For this review, take the finished solid that the model builds, in its own axes (mm). Face numbers are marked on the shaded views. A direction names the side the tool comes from. Round coordinates to 2 decimals unless told otherwise and drop trailing zeros. Order: outer loops, then holes, each group sorted by start corner. A loop starts at its lowest first (then second) coordinate and runs counter-clockwise, first axis right, second up.
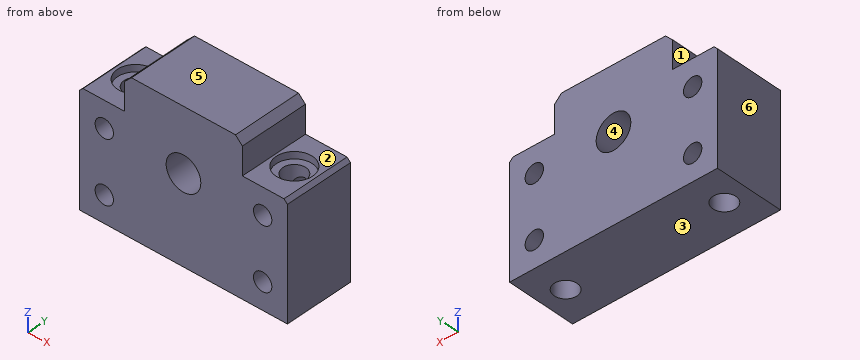
from build123d import *

# Parameters (mm, degrees)
F0_R     = 2.65
F0_R_2   = 5
F1_DEPTH = 10
F2_SIZE  = 1
F3_SIZE  = 2
F4_R     = 3.3
F5_DEPTH = 33
F4_R_2   = 5.25
F6_DEPTH = 2


with BuildPart() as f1:
    # F0 (on Front) → F1 (new body, symmetric)
    with BuildSketch(Plane.XZ):
        Polygon((17, 18), (0, 18), (-17, 18), (-17, 8), (-30, 8), (-30, -25), (0, -25), (30, -25), (30, 8), (17, 8), align=None)
        with Locations((-22.85, -17.35)):
            Circle(F0_R, mode=Mode.SUBTRACT)
        with Locations((22.85, -17.35)):
            Circle(F0_R, mode=Mode.SUBTRACT)
        with Locations((-22.85, 0.45)):
            Circle(F0_R, mode=Mode.SUBTRACT)
        Circle(F0_R_2, mode=Mode.SUBTRACT)
        with Locations((22.85, 0.45)):
            Circle(F0_R, mode=Mode.SUBTRACT)
    extrude(amount=F1_DEPTH, both=True)

    # F2
    f2_edges = [f1.edges().sort_by_distance(p)[0] for p in [
        (30, 0, 8),
        (-30, 0, 8),
    ]]
    chamfer(f2_edges, length=F2_SIZE)

    # F3
    f3_edges = [f1.edges().sort_by_distance(p)[0] for p in [
        (17, 0, 18),
        (-17, 0, 18),
    ]]
    chamfer(f3_edges, length=F3_SIZE)

    # F4 (on face) → F5 (cut, through all)
    with BuildSketch(Plane.XY.offset(8)):
        with Locations((-22.9, 0)):
            Circle(F4_R)
        with Locations((22.9, 0)):
            Circle(F4_R)
    extrude(amount=-F5_DEPTH, mode=Mode.SUBTRACT)

    # F4 (on face) → F6 (cut)
    with BuildSketch(Plane.XY.offset(8)):
        with Locations((22.9, 0)):
            Circle(F4_R_2)
        with Locations((22.9, 0)):
            Circle(F4_R, mode=Mode.SUBTRACT)
        with Locations((-22.9, 0)):
            Circle(F4_R_2)
        with Locations((-22.9, 0)):
            Circle(F4_R, mode=Mode.SUBTRACT)
    extrude(amount=-F6_DEPTH, mode=Mode.SUBTRACT)


solid = f1.part
(1) Add section A-A on y = 0. Count the separate pieces of the cut face and the enclosed holes in it, plus the area to 3 significant figures.
(2) Add section D-D on y = -8.5. Give the boundary of the cut face in (x, z), plus the area to 3 significant figures.
(3) Wall thickness on L1, parallel to Y at x = -22.9, z = 7.45; L2, parallel to X at y = -4.25, z = -17.35; L3, parallel to Z at x = 21.5, y = 7.75: over which ranges is each line inside the solid? List them lowest first.
(4) Clearance check with flat-ended pins moving along their axes: P1, Ø4, axis at y = -1.5, z = 10.5, coming from the +X side; P2, Ø4, axis at y = 3.5, z = 11, coming from the -X side; P3, Ø6, axis at x = 22.5, y = 1, coming from the +Z side; P4, Ø4, axis at x = -22.85, z = 0.45, coming from the -Y side. State where each tip first meets the part, or that it passes through.
(5) Add section C-C on z = -17.35. Give the boundary of the cut face in (x, y).
(6) Tool access review of the marked faces 1, 2 and 3: name each direction out of +Z, -Z, +X, -X, +Y, -Y from which nothing blocks a thin tool from reaching the whole face with its end or side.
(7) Add section B-B on x = 3. Give the boundary of the cut face in (y, z).
(8) Draft analysis for pull direction Z (two halves, no side actions). For the marked faces 4, 5 and 6, state which applies: pulls with the +Z half, pulls with the -Z half, needs draft (parallel to the pull), parting line crosses it, or undercut.
Here are the results:
1. separate pieces: 3
1. enclosed holes: 1
1. area: 1,790 mm2
2. outline: (-30, -25) - (30, -25) - (30, 7) - (29, 8) - (17, 8) - (17, 16) - (15, 18) - (-15, 18) - (-17, 16) - (-17, 8) - (-29, 8) - (-30, 7) - close; hole circle Ø5.3 at (-22.85, -17.35); hole circle Ø5.3 at (-22.85, 0.45); hole circle Ø10 at (0, 0); hole circle Ø5.3 at (22.85, -17.35); hole circle Ø5.3 at (22.85, 0.45)
2. area: 2,150 mm2
3. L1: y = -10 to -5.25, 5.25 to 10
3. L2: x = -30 to -25.5, -20.2 to 20.2, 25.5 to 30
3. L3: z = -25 to -19.63, -15.07 to -1.83, 2.73 to 8
4. P1: stops at x = 17
4. P2: stops at x = -17
4. P3: stops at z = 6
4. P4: passes through
5. outline: (-30, -10) - (-25.5, -10) - (-25.5, -2.03) arc R3.3 cw to (-25.5, 2.03) - (-25.5, 10) - (-30, 10) - close; (-20.2, -10) - (20.2, -10) - (20.2, -1.9) arc R3.3 cw to (20.2, 1.9) - (20.2, 10) - (-20.2, 10) - (-20.2, 1.9) arc R3.3 cw to (-20.2, -1.9) - close; (25.5, -10) - (30, -10) - (30, 10) - (25.5, 10) - (25.5, 2.03) arc R3.3 cw to (25.5, -2.03) - close
6. face 1: +Z, -X, +Y, -Y
6. face 2: +Z, +X, +Y, -Y
6. face 3: -Z, +X, -X, +Y, -Y
7. outline: (-10, -25) - (10, -25) - (10, -4) - (-10, -4) - close; (-10, 4) - (10, 4) - (10, 18) - (-10, 18) - close
8. face 4: undercut
8. face 5: pulls with the +Z half
8. face 6: needs draft
